```python
from build123d import *

# Parameters (mm, degrees)
F0_W     = 38.1
F0_H     = 38.1
F0_W_2   = 31.75
F0_H_2   = 31.75
F1_DEPTH = 63.5
F3_DEPTH = 38.101


with BuildPart() as f1:
    # F0 (on Top) → F1 (new body)
    with BuildSketch(Plane.XY):
        Rectangle(F0_W, F0_H)
        Rectangle(F0_W_2, F0_H_2, mode=Mode.SUBTRACT)
    extrude(amount=F1_DEPTH)

    # F2 (on face) → F3 (cut, through all)
    with BuildSketch(Plane.XZ.offset(19.05)):
        with BuildLine():
            ThreePointArc((3.175, 31.75), (1.564319, 34.512885), (-1.633524, 34.47254))
            Line((-1.633524, 34.47254), (1.633524, 29.02746))
            ThreePointArc((1.633524, 29.02746), (2.762885, 30.185681), (3.175, 31.75))
        make_face()
        with BuildLine():
            Line((1.633524, 29.02746), (-1.633524, 34.47254))
            ThreePointArc((-1.633524, 34.47254), (-2.72254, 30.116476), (1.633524, 29.02746))
        make_face()
    extrude(amount=-F3_DEPTH, mode=Mode.SUBTRACT)


solid = f1.part
```
Build history of the part. All positions in model axes, mm. A direction names the side the tool comes from. Coordinates: 2 decimals unless noted, no trailing zeros. Write each loop counter-clockwise with the first axis right and the second up, starting at its lowest first coordinate (ties: lowest second). Pieces come first, ordered by that corner, then holes.
1. Band-saw the part on A-A, the plane x = -7. Give the cut face in (y, z) (3 decimals).
Answer block:
outline: (-19.05, 0) - (-15.875, 0) - (-15.875, 63.5) - (-19.05, 63.5) - close; (15.875, 0) - (19.05, 0) - (19.05, 63.5) - (15.875, 63.5) - close
2. 3-axis set-ups, long thin cutter, end or side, ignore diameter. For faces 1 (the flat face through (-15.875, 0, 31)), 2 (the flat face through (19.05, 0, 31)): which of +Z, -Z, +X, -X, +Y, -Y reach the whole face in a straight line?
Answer block:
face 1: +Z, -Z
face 2: +Z, -Z, +X, +Y, -Y
3. Pull direction X, two halves, no side cores. Call faces 3 (the flat face through (-19.05, 0, 31)), 4 (the flat face through (15.875, 0, 31)), 5 (the flat face through (4, 19.05, 31)): released by +X, released by -X, zero draft, split by the parting line, or undercut.
Answer block:
face 3: released by -X
face 4: undercut
face 5: zero draft
4. Drop a flat-ended pin along its axis: pin 1 (3 mm diameter, centred on x = 14, y = -13, fed in from -Z). Give the stop position or say it passes through.
Answer block:
pin 1: passes through
5. Drill centre line: probe 1 along X at (y, z) = (-7.5, 59) (3 decimals). Where is it in solid material? Low to high.
Answer block:
probe 1: x = -19.05 to -15.875, 15.875 to 19.05
6. Band-saw the part on C-C, the plane x = 0. Give the cut face in (y, z) (3 decimals).
Answer block:
outline: (-19.05, 0) - (-15.875, 0) - (-15.875, 28.575) - (-19.05, 28.575) - close; (-19.05, 34.925) - (-15.875, 34.925) - (-15.875, 63.5) - (-19.05, 63.5) - close; (15.875, 0) - (19.05, 0) - (19.05, 28.575) - (15.875, 28.575) - close; (15.875, 34.925) - (19.05, 34.925) - (19.05, 63.5) - (15.875, 63.5) - close
